Input: part model. Units: mm. Frame: model coordinates. A direction names the side the tool comes from. Coordinates: 2 decimals unless noted, no trailing zeros. Put each result on its own line as item: value. Start each with the question number.
1. Line query: line 1 (X direction, y = -133.5, z = -6); line 2 (Z direction, x = 2, y = -127); line 3 (X direction, y = -110, z = -3). Output: solid intervals per line, ascending.
2. Pull-direction query (Y, two-part tool) for faces 4 (the flat face through (-33, 51.119, 0)), 5 (the flat face through (-34, -195.881, 0)), 6 (the cylindrical face through (-63.24, -191.32, -9.46)), 7 (the cylindrical face through (-31.54, 32.36, -7.44)); classes: released by +Y, released by -Y, zero draft, split by the parting line, or undercut.
3. Pin query (flat end, axial travel): pin 1 (10 mm diameter, centred on x = -58, z = -48.5, fed in from +Y); pin 2 (2 mm diameter, centred on x = -75.5, z = 9, fed in from -Y); pin 3 (4 mm diameter, centred on x = -34.5, y = 42, fed in from +Z). Return the tip coordinate at first contact, or that it passes through.
4. Access query for faces 1 (the flat face through (-41, 14.119, 0)), 2 (the flat face through (-33, 41, 37)), 3 (the cylindrical face through (-39.316, 38.825, 20.328)). Directions: +Z, -Z, +X, -X, +Y, -Y. A direction counts if a zero-diameter tool reaches every point of the face in a straight line with its end or side. Return the directions, or none.
from build123d import *

# Parameters (mm, degrees)
SKETCH2_R           = 7.621417702
BOSS_EXTRUDE1_DEPTH = 37
SKETCH3_R           = 6.301348683
BOSS_EXTRUDE2_DEPTH = 37


with BuildPart() as part:
    # Sketch1 → Revolve1 (revolve)
    with BuildSketch(Plane.XY, mode=Mode.PRIVATE) as revolve1_sk:
        with BuildLine():
            Line((-13.94213087, 14.118857143), (-33.19213087, 14.118857143))
            Line((-33.19213087, 14.118857143), (-33.19213087, 5.118857143))
            Line((-33.19213087, 5.118857143), (-33.19213087, -186.881142857))
            Line((-33.19213087, -186.881142857), (-33.19213087, -195.881142857))
            Line((-33.19213087, -195.881142857), (-1.69213087, -195.881142857))
            Line((-1.69213087, -195.881142857), (-1.69213087, -186.881142857))
            ThreePointArc((-1.69213087, -186.881142857), (29.176808752, -88.520852439), (-13.94213087, 5.118857143))
            Line((-13.94213087, 5.118857143), (-13.94213087, 14.118857143))
        make_face()
    revolve(revolve1_sk.sketch.rotate(Axis((-33.19213087, 5.118857143, 0), (0, -1, 0)), 180), axis=Axis((-33.19213087, 5.118857143, 0), (0, -1, 0)))

    # Sketch2 → Boss-Extrude1 (add)
    with BuildSketch(Plane(origin=(0, 14.118857143, 0), x_dir=(1, 0, 0), z_dir=(0, 1, 0))):
        with Locations(Location((-33.19213087, 0, 0), (0, 0, 180))):
            Circle(SKETCH2_R)
    extrude(amount=BOSS_EXTRUDE1_DEPTH)

    # Sketch3 → Boss-Extrude2 (add)
    with BuildSketch(Plane.XY):
        with Locations(Location((-33.305381498, 40.717884654, 0), (0, 0, 180))):
            Circle(SKETCH3_R)
    extrude(amount=BOSS_EXTRUDE2_DEPTH)


solid = part.part
Report:
1. line 1: x = -90.99 to 24.6
1. line 2: z = -48.13 to 48.13
1. line 3: x = -95.25 to 28.86
2. face 4: released by +Y
2. face 5: released by -Y
2. face 6: zero draft
2. face 7: undercut
3. pin 1: stops at y = -37.6
3. pin 2: stops at y = -171.36
3. pin 3: stops at z = 37
4. face 1: none
4. face 2: +Z, +X, -X, +Y
4. face 3: +Z
